Check sheet for the modelled part. Datum: model origin and axes. Units: mm. Give positions to 0.01 mm unless a question says otherwise; leave off trailing zeros. Write each loop counter-clockwise with the first axis right and the second up, starting at its lowest first coordinate (ties: lowest second). Pieces come first, ordered by that corner, then holes. Notation, with made-up numbers: M 83,89 L 95,89 A14 cw 95,93 Z; hole C 67.25,57.25 d1. An arc over 180 degrees is marked long. One line per item, written item: value. Start each with the question number.
from build123d import *

# Parameters (mm, degrees)
BOSS_EXTRUDE1_DEPTH = 2
SKETCH1_3_W         = 37.4
SKETCH1_3_H         = 6
SKETCH1_3_W_2       = 13.3
SKETCH1_3_H_2       = 5
SKETCH1_3_W_3       = 12
SKETCH1_3_H_3       = 30
BOSS_EXTRUDE2_DEPTH = 20


with BuildPart() as part:
    # Sketch1 → Boss-Extrude1 (new body)
    with BuildSketch(Plane.XY):
        with BuildLine():
            Line((4, 0), (64, 0))
            ThreePointArc((64, 0), (66.828427125, 1.171572875), (68, 4))
            Line((68, 4), (68, 76.8))
            ThreePointArc((68, 76.8), (66.828427125, 79.628427125), (64, 80.8))
            Line((64, 80.8), (4, 80.8))
            ThreePointArc((4, 80.8), (1.171572875, 79.628427125), (0, 76.8))
            Line((0, 76.8), (0, 4))
            ThreePointArc((0, 4), (1.171572875, 1.171572875), (4, 0))
        make_face()
    extrude(amount=BOSS_EXTRUDE1_DEPTH)

    # Sketch1<3> → Boss-Extrude2 (add)
    with BuildSketch(Plane.XY):
        with BuildLine():
            ThreePointArc((0, 4), (1.171572875, 1.171572875), (4, 0))
            Line((4, 0), (64, 0))
            ThreePointArc((64, 0), (66.828427125, 1.171572875), (68, 4))
            Line((68, 4), (68, 76.8))
            ThreePointArc((68, 76.8), (66.828427125, 79.628427125), (64, 80.8))
            Line((64, 80.8), (4, 80.8))
            ThreePointArc((4, 80.8), (1.171572875, 79.628427125), (0, 76.8))
            Line((0, 76.8), (0, 4))
        make_face()
        with Locations((22.7, 7.8)):
            Rectangle(SKETCH1_3_W, SKETCH1_3_H, mode=Mode.SUBTRACT)
        with Locations((57.35, 7.5)):
            Rectangle(SKETCH1_3_W_2, SKETCH1_3_H_2, mode=Mode.SUBTRACT)
        with Locations((22.7, 15.8)):
            Rectangle(SKETCH1_3_W, SKETCH1_3_H, mode=Mode.SUBTRACT)
        with Locations((22.7, 23.8)):
            Rectangle(SKETCH1_3_W, SKETCH1_3_H, mode=Mode.SUBTRACT)
        with Locations((22.7, 31.8)):
            Rectangle(SKETCH1_3_W, SKETCH1_3_H, mode=Mode.SUBTRACT)
        with Locations((22.7, 39.8)):
            Rectangle(SKETCH1_3_W, SKETCH1_3_H, mode=Mode.SUBTRACT)
        with Locations((10, 61.8)):
            Rectangle(SKETCH1_3_W_3, SKETCH1_3_H_3, mode=Mode.SUBTRACT)
        with Locations((26, 61.8)):
            Rectangle(SKETCH1_3_W_3, SKETCH1_3_H_3, mode=Mode.SUBTRACT)
        with Locations((57.35, 15.7)):
            Rectangle(SKETCH1_3_W_2, SKETCH1_3_H_2, mode=Mode.SUBTRACT)
        with Locations((57.35, 32.1)):
            Rectangle(SKETCH1_3_W_2, SKETCH1_3_H_2, mode=Mode.SUBTRACT)
        with Locations((57.35, 23.9)):
            Rectangle(SKETCH1_3_W_2, SKETCH1_3_H_2, mode=Mode.SUBTRACT)
        with Locations((57.35, 40.3)):
            Rectangle(SKETCH1_3_W_2, SKETCH1_3_H_2, mode=Mode.SUBTRACT)
        with Locations((42, 61.8)):
            Rectangle(SKETCH1_3_W_3, SKETCH1_3_H_3, mode=Mode.SUBTRACT)
        with Locations((58, 61.8)):
            Rectangle(SKETCH1_3_W_3, SKETCH1_3_H_3, mode=Mode.SUBTRACT)
    extrude(amount=BOSS_EXTRUDE2_DEPTH)


solid = part.part
1) Cross-section at D-D (x = 33.5). Record the boundary of the cut face in (y, z), plus the area to 3 significant figures.
2) Material ranges on L1, parallel to X at y = 54, z = 12.25; L2, parallel to X at y = 34, z = 10.75; L3, parallel to Z at x = 26.5, y = 8, recorded low to high. Write a range as from..to.
3) Draft check along Y on faces 1 (the flat face through (68, 40, 10)), 2 (the flat face through (64, 32, 11)). Enter one of: released by +Y, released by -Y, zero draft, split by the parting line, or undercut.
4) Cross-section at B-B (y = 24). Record the boundary of the cut face in (x, z).
5) Cross-section at C-C (z = 6.25). State how many separate pieces and enclosed holes the cut face has, plus the area to 3 significant figures.
6) Cross-section at A-A (x = 55.5). Record the boundary of the cut face in (y, z).
7) Gauge pin test, flat ends, axial feed: pin 1 (1.8 mm diameter, centred on x = 20.5, y = 8.5, fed in from +Z); pin 2 (5.5 mm diameter, centred on x = 54.5, y = 7, fed in from +Z). Record the tip position at first contact, or that the pin passes through.
Data:
1. outline: M 0,0 L 80.8,0 L 80.8,20 L 42.8,20 L 42.8,2 L 36.8,2 L 36.8,20 L 34.8,20 L 34.8,2 L 28.8,2 L 28.8,20 L 26.8,20 L 26.8,2 L 20.8,2 L 20.8,20 L 18.8,20 L 18.8,2 L 12.8,2 L 12.8,20 L 10.8,20 L 10.8,2 L 4.8,2 L 4.8,20 L 0,20 Z
1. area: 1,080 mm2
2. L1: x = 0..4, 16..20, 32..36, 48..52, 64..68
2. L2: x = 0..4, 41.4..50.7, 64..68
2. L3: z = 0..2
3. face 1: zero draft
3. face 2: undercut
4. outline: M 0,0 L 68,0 L 68,20 L 64,20 L 64,2 L 50.7,2 L 50.7,20 L 41.4,20 L 41.4,2 L 4,2 L 4,20 L 0,20 Z
5. separate pieces: 1
5. enclosed holes: 14
5. area: 2,590 mm2
6. outline: M 0,0 L 80.8,0 L 80.8,20 L 76.8,20 L 76.8,2 L 46.8,2 L 46.8,20 L 42.8,20 L 42.8,2 L 37.8,2 L 37.8,20 L 34.6,20 L 34.6,2 L 29.6,2 L 29.6,20 L 26.4,20 L 26.4,2 L 21.4,2 L 21.4,20 L 18.2,20 L 18.2,2 L 13.2,2 L 13.2,20 L 10,20 L 10,2 L 5,2 L 5,20 L 0,20 Z
7. pin 1: stops at z = 2
7. pin 2: stops at z = 20
